from build123d import *

# Parameters (mm, degrees)
SKETCH1_W               = 20
SKETCH1_H               = 10.2
BOSS_EXTRUDE1_DEPTH     = 3.2
CUT_EXTRUDE1_DEPTH      = 12.67261753
CUT_EXTRUDE1_DEPTH_BACK = 12.67261753
SKETCH2_R               = 1.25
SKETCH3_W               = 3.3
SKETCH3_H               = 0.4
BOSS_EXTRUDE2_DEPTH     = 3.5


with BuildPart() as part:
    # Sketch1 → Boss-Extrude1 (new, symmetric)
    with BuildSketch(Plane(origin=(0, 0, 0), x_dir=(0, 0, -1), z_dir=(1, 0, 0))):
        Rectangle(SKETCH1_W, SKETCH1_H)
    extrude(amount=BOSS_EXTRUDE1_DEPTH, both=True)

    # Sketch2 → Cut-Extrude1 (cut, two sides: drawn at the far end of the back side and taken through both)
    with BuildSketch(Plane(origin=(0, 0, 0), x_dir=(0, 0, -1), z_dir=(1, 0, 0)).offset(-CUT_EXTRUDE1_DEPTH_BACK)):
        with Locations((-5, -2.2)):
            Circle(SKETCH2_R)
        with Locations((4.5, -2.2)):
            Circle(SKETCH2_R)
    extrude(amount=CUT_EXTRUDE1_DEPTH + CUT_EXTRUDE1_DEPTH_BACK, mode=Mode.SUBTRACT)

    # Sketch3 → Boss-Extrude2 (add)
    with BuildSketch(Plane.XZ.offset(5.1)):
        with Locations((0, -8.4)):
            Rectangle(SKETCH3_W, SKETCH3_H)
        with Locations((0, 0.4)):
            Rectangle(SKETCH3_W, SKETCH3_H)
        with Locations((0, 7.7)):
            Rectangle(SKETCH3_W, SKETCH3_H)
    extrude(amount=BOSS_EXTRUDE2_DEPTH)


solid = part.part
Design review of the part built by this model. Coordinates are the model's own, in mm. A direction names the side the tool comes from. Round coordinates to 2 decimals unless told otherwise and drop trailing zeros. Write each loop counter-clockwise with the first axis right and the second up, starting at its lowest first coordinate (ties: lowest second). Pieces come first, ordered by that corner, then holes. Notation, with made-up numbers: M -4,21.25 L 3,21.25 A11 cw 3,35.25 Z; hole C 49.25,9 d10. An arc over 180 degrees is marked long. One line per item, written item: value. Start each with the question number.
1. Take a section at D-D on z = 5. State the section outline as (x, y) points.
2. Take a section at C-C on z = -3.5. State the section outline as (x, y) points, then the cut area to 3 significant figures.
3. For faces 1 (the face through (0, -7, -8.2)), 2 (the face through (0, -7, -8.6)), 3 (the face through (0, -7, 7.9)), 4 (the face through (0, 0, -10)), 5 (the face through (0, 0, 10)), list the 3-axis set-ups (+Z, -Z, +X, -X, +Y, -Y) from which the entire face can be reached by the end or side of a thin tool; tool diameter is ignored.
4. Take a section at A-A on y = -2.2. State the section outline as (x, z) points.
5. Take a section at B-B on x = -1. State the section outline as (y, z) points, then the cut area to 3 significant figures.
6. Draft analysis for pull direction Y (two halves, no side actions). For faces 6 (the face through (0, 5.1, 0)), 7 (the face through (-0.04, -3.42, -4.23)), 8 (the face through (-3.2, 0, 0)), state which applies: pulls with the +Y half, pulls with the -Y half, needs draft (parallel to the pull), parting line crosses it, or undercut.
7. Clearance check with flat-ended pins moving along their axes: P1, Ø3.5, axis at x = 0, y = -7.5, coming from the +Z side; P2, Ø1, axis at x = 2.5, y = -6, coming from the +Z side; P3, Ø2.5, axis at x = 0, y = -7.5, coming from the -Z side. State where each tip first meets the part, or that it passes through.
8. To check wall thickness, follow probe 1 along Z at (x, y) = (-1.25, -2.2); probe 2 along Z at (x, y) = (0.25, -7.25); probe 3 along Y at (x, z) = (-1.5, -4.5). State the ranges of each line that lie inside material, in increasing order. Write a range as from..to.
Computed:
1. outline: M -3.2,-5.1 L 3.2,-5.1 L 3.2,-3.45 L -3.2,-3.45 Z; M -3.2,-0.95 L 3.2,-0.95 L 3.2,5.1 L -3.2,5.1 Z
2. outline: M -3.2,-5.1 L 3.2,-5.1 L 3.2,-2.95 L -3.2,-2.95 Z; M -3.2,-1.45 L 3.2,-1.45 L 3.2,5.1 L -3.2,5.1 Z
2. area: 55.7 mm²
3. face 1: +X, -X, -Y
3. face 2: -Z, +X, -X, -Y
3. face 3: +Z, +X, -X, -Y
3. face 4: -Z, +X, -X, +Y, -Y
3. face 5: +Z, +X, -X, +Y, -Y
4. outline: M -3.2,-10 L 3.2,-10 L 3.2,-5.75 L -3.2,-5.75 Z; M -3.2,-3.25 L 3.2,-3.25 L 3.2,3.75 L -3.2,3.75 Z; M -3.2,6.25 L 3.2,6.25 L 3.2,10 L -3.2,10 Z
5. outline: M -8.6,-8.6 L -5.1,-8.6 L -5.1,-10 L 5.1,-10 L 5.1,10 L -5.1,10 L -5.1,7.9 L -8.6,7.9 L -8.6,7.5 L -5.1,7.5 L -5.1,0.6 L -8.6,0.6 L -8.6,0.2 L -5.1,0.2 L -5.1,-8.2 L -8.6,-8.2 Z; hole C -2.2,-4.5 d2.5; hole C -2.2,5 d2.5
5. area: 198 mm²
6. face 6: pulls with the +Y half
6. face 7: undercut
6. face 8: needs draft
7. P1: stops at z = 7.9
7. P2: passes through
7. P3: stops at z = -8.6
8. probe 1: z = -10..-5.75, -3.25..3.75, 6.25..10
8. probe 2: z = -8.6..-8.2, 0.2..0.6, 7.5..7.9
8. probe 3: y = -5.1..-3.45, -0.95..5.1
